Can you work these out from the drawing? Everything is in mm from the part's minimum corner. A direction names the side the tool comes from. Give positions to 0.01 mm unless a question says otherwise; leave off trailing zeros. Write each loop counter-clockwise with the first axis right and the second up, starting at its lowest first coordinate (ties: lowest second). Pieces come first, ordered by that corner, then holes. Notation, with made-up numbers: M -19.75,10.5 L 39.25,10.5 A23 cw 39.25,37.5 Z; hole C 63.5,-6 d3. An arc over 180 degrees is marked long. One line per item, written item: value.
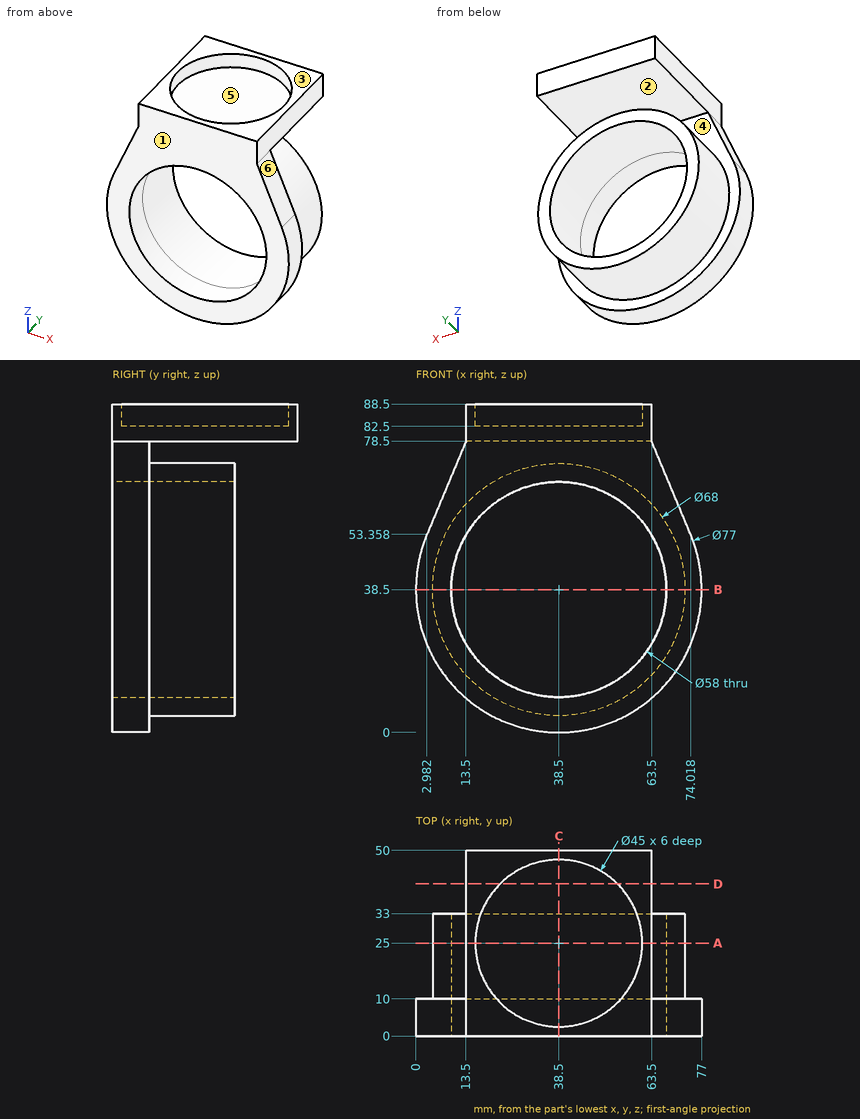
1) I'm going to push flat-ended pins straight in: pin 1 (10 mm diameter, centred on x = 39.5, y = 43, fed in from +Z); pin 2 (13.5 mm diameter, centred on x = 27.5, y = 28.5, fed in from +Z); pin 3 (5 mm diameter, centred on y = 29.5, z = 43.5, fed in from -X); pin 4 (11 mm diameter, centred on y = 16, z = 85, fed in from -X). Where does each tip first touch, or does it pass through?
Outcome:
pin 1: stops at z = 88.5
pin 2: stops at z = 82.5
pin 3: stops at x = 4.59
pin 4: stops at x = 13.5
2) If we section it at C-C, the plane x = 38.5: Write out the boundary of the cut face in (y, z), then the cut area to 3 significant figures.
Outcome:
outline: M 0,0 L 10,0 L 10,4.5 L 33,4.5 L 33,9.5 L 0,9.5 Z; M 0,67.5 L 33,67.5 L 33,72.5 L 10,72.5 L 10,78.5 L 50,78.5 L 50,88.5 L 47.5,88.5 L 47.5,82.5 L 2.5,82.5 L 2.5,88.5 L 0,88.5 Z
area: 665 mm^2
3) We'd pull the mould along Z, two halves only. Please class the marked faces 1, 2 and 3: pulls with the +Z half, pulls with the -Z half, needs draft (parallel to the pull), parting line crosses it, or undercut.
Outcome:
face 1: needs draft
face 2: undercut
face 3: pulls with the +Z half
4) If we section it at B-B, the plane z = 38.5: Write out the boundary of the cut face in (x, y), then the cut area to 3 significant figures.
Outcome:
outline: M 0,0 L 9.5,0 L 9.5,33 L 4.5,33 L 4.5,10 L 0,10 Z; M 67.5,0 L 77,0 L 77,10 L 72.5,10 L 72.5,33 L 67.5,33 Z
area: 420 mm^2
5) Please list where these lines run through material, in increasing order: L1, parallel to X at y = 24.75, z = 38.5; L2, parallel to Z at x = 45, y = 17.5; L3, parallel to Z at x = 38, y = 6 (1 decimal). Write a range as from..to.
Outcome:
L1: x = 4.5..9.5, 67.5..72.5
L2: z = 5.13..10.24, 66.76..71.87, 78.5..82.5
L3: z = 0..9.5, 67.5..82.5
6) If we section it at D-D, the plane y = 41: Write out the boundary of the cut face in (x, z).
Outcome:
outline: M 13.5,78.5 L 63.5,78.5 L 63.5,88.5 L 54.32,88.5 L 54.32,82.5 L 22.68,82.5 L 22.68,88.5 L 13.5,88.5 Z
7) If we section it at A-A, the plane y = 25: Write out the boundary of the cut face in (x, z).
Outcome:
outline: C 38.5,38.5 d68; M 13.5,78.5 L 63.5,78.5 L 63.5,88.5 L 61,88.5 L 61,82.5 L 16,82.5 L 16,88.5 L 13.5,88.5 Z; hole C 38.5,38.5 d58
8) On a 3-axis mill with a long thin cutter (end or side, diameter ignored), from which of +Z, -Z, +X, -X, +Y, -Y can I reach the whole of each face in a straight line? I mean the marked faces 4, 5 and 6. Say none if no direction works.
Outcome:
face 4: +Y
face 5: +Z
face 6: +Z, +X, +Y, -Y
